Could you check a few things on this drawing? It's one solid part, dimensions in mm from its lowest x, y, z. A direction names the side the tool comes from. Give positions to 0.01 mm unless a question says otherwise; leave off trailing zeros. Write each loop counter-clockwise with the first axis right and the second up, starting at its lowest first coordinate (ties: lowest second). Pieces come first, ordered by that corner, then holes.
1. Suppose I cut it at C-C (y = 1.25). Please give me the cut outline in (x, z).
2. Suppose I cut it at D-D (y = 10). Please give me the cut outline in (x, z), and give its area (3 significant figures).
3. On a 3-axis mill with a long thin cutter (end or side, diameter ignored), from which of +Z, -Z, +X, -X, +Y, -Y can I reach the whole of each face in a straight line? I mean the marked faces 1, 2, 3, 4 and 5. Say none if no direction works.
4. Suppose I cut it at B-B (y = 5.75). Please give me the cut outline in (x, z).
5. I'm going to push flat-ended pins straight in: pin 1 (3 mm diameter, centred on y = 10.5, z = 6.5, fed in from -X); pin 2 (1 mm diameter, centred on x = 2.5, z = 6, fed in from +Y); pin 3 (3.5 mm diameter, centred on y = 6, z = 5, fed in from -X). Where does each tip first touch, or does it pass through?
6. Suppose I cut it at A-A (z = 1). Please give me the cut outline in (x, y), and give its area (3 significant figures).
7. If I drill on probe 1 along Y at (x, z) = (5.5, 5); probe 2 along Z at (x, y) = (7, 2.5); probe 3 along X at (y, z) = (5, 4.5), over which ranges is the centre line in solid material (lowest first)?
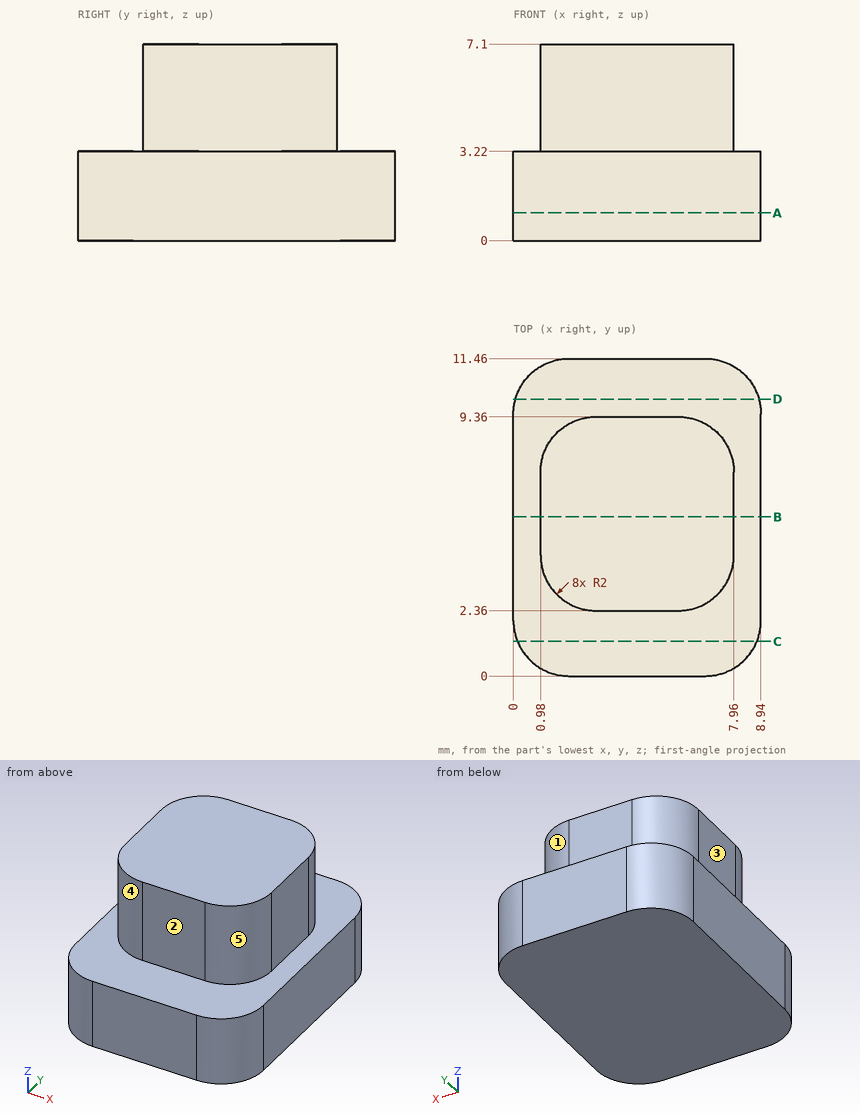
Checks:
1. outline: (0.15, 0) - (8.79, 0) - (8.79, 3.22) - (0.15, 3.22) - close
2. outline: (0.07, 0) - (8.87, 0) - (8.87, 3.22) - (0.07, 3.22) - close
2. area: 28.3 mm2
3. face 1: +Z, +X, +Y
3. face 2: +Z, +X, -X, -Y
3. face 3: +Z, -X, +Y, -Y
3. face 4: +Z, -X, -Y
3. face 5: +Z, +X, -Y
4. outline: (0, 0) - (8.94, 0) - (8.94, 3.22) - (7.96, 3.22) - (7.96, 7.1) - (0.98, 7.1) - (0.98, 3.22) - (0, 3.22) - close
5. pin 1: stops at x = 1.84
5. pin 2: stops at y = 9.36
5. pin 3: stops at x = 0.98
6. outline: (0, 2) arc R2 ccw to (2, 0) - (6.94, 0) arc R2 ccw to (8.94, 2) - (8.94, 9.46) arc R2 ccw to (6.94, 11.46) - (2, 11.46) arc R2 ccw to (0, 9.46) - close
6. area: 99.0 mm2
7. probe 1: y = 2.36 to 9.36
7. probe 2: z = 0 to 3.22
7. probe 3: x = 0.98 to 7.96
